The model under review builds one solid part; all positions refer to its coordinate system, in mm. A direction names the side the tool comes from. Coordinates: 2 decimals unless noted, no trailing zeros. Order: outer loops, then holes, each group sorted by start corner. A loop starts at its lowest first (then second) coordinate and runs counter-clockwise, first axis right, second up.
Autodesk Inventor part; units mm, degrees
ref_plane "YZ Plane" through (0, 0, 0) normal (1, 0, 0) x (0, 1, 0)
ref_plane "XZ Plane" through (0, 0, 0) normal (0, 1, 0) x (-1, 0, 0)
ref_plane "XY Plane" through (0, 0, 0) normal (0, 0, 1) x (1, 0, 0)
sketch "Náčrt1" plane through (0, 0, 0) normal (0, 0, 1) x (1, 0, 0)
  line L0 (-25, 0) -> (25, 0) construction
  line L1 (-25, -5) -> (25, -5)
  line L2 (25, 5) -> (-25, 5)
  arc A0 (-25, 5) -> (-25, -5) centre (-25, 0) ccw
  arc A1 (25, -5) -> (25, 5) centre (25, 0) ccw
  point P0 (0, 0)
  point P1 (30, 0)
  dimension "d0" = 30
  dimension "d1" = 5
extrude "Vysunutí1" add sketch "Náčrt1" along normal blind 0.5
sketch "Náčrt2" plane through (0, 0, 0) normal (0, 0, -1) x (-1, 0, 0)
  arc A0 (25, -5) -> (25, 5) centre (25, 0) ccw
  circle A1 centre (25, 0) radius 2
  point P0 (0, 0)
  dimension "d4" = 4
extrude "Vysunutí2" cut sketch "Náčrt2" against normal through all
pattern_linear "Obdélníkové pole1" count 7 spacing 10 along (1, 0, 0) of "Vysunutí2"
sketch "Náčrt3" plane through (0, 0, 0.5) normal (0, 0, 1) x (1, 0, 0)
  circle A0 centre (-15, 0) radius 2
  line L0 (-15, 2) -> (14.9898, 2)
  line L1 (14.9898, 2) -> (14.9898, -2)
  line L2 (14.9898, -2) -> (-15, -2)
  point P0 (0, 0)
extrude "Vysunutí3" cut sketch "Náčrt3" against normal blind 10 contours A0 L0 L1 L2
properties part number "2006"
(1) Consider section A-A (y = 0). Give the boundary of the cut face in (x, z), then the cut area to 3 significant figures.
(2) Tool access review of faces 5 (the face through (-0.4, 2.3, 0)), 6 (the face through (17, 0, 0.2)): name each direction out of +Z, -Z, +X, -X, +Y, -Y from which nothing blocks a thin tool from reaching the whole face with its end or side.
(3) Consider section B-B (z = 0.1). Give the number of separate pieces and of enclosed holes in the cut face, then the cut area to 3 significant figures.
(4) Wall thickness on line 1 (Y direction, x = -25, z = 0.45); line 2 (X direction, y = -0.25, z = 0.15); line 3 (X direction, y = -1.75, z = 0.4): over which ranges is each line inside the solid? List them lowest first.
(5) The part is to be moulded in two halves that separate along Y. For faces 1 (the face through (-17, 0, 0.2)), 2 (the face through (26.998, 0.088, 0.246)), 3 (the face through (-0.4, 2.3, 0.5)), 4 (the face through (-30, -0.1, 0.2)), say which applies: +Y half, -Y half, draft (parallel to the pull), parting line (faces both ways), or undercut.
(6) Consider section C-C (x = -4.5). Give the boundary of the cut face in (y, z).
(7) Consider section D-D (y = 3). Give the boundary of the cut face in (x, z), then the cut area to 3 significant figures.
Findings:
1. outline: (-30, 0) - (-27, 0) - (-27, 0.5) - (-30, 0.5) - close; (-23, 0) - (-17, 0) - (-17, 0.5) - (-23, 0.5) - close; (17, 0) - (23, 0) - (23, 0.5) - (17, 0.5) - close; (27, 0) - (30, 0) - (30, 0.5) - (27, 0.5) - close
1. area: 9.00 mm2
2. face 5: -Z, +X, -X, +Y, -Y
2. face 6: +Z, -Z
3. separate pieces: 1
3. enclosed holes: 3
3. area: 421 mm2
4. line 1: y = -5 to -2, 2 to 5
4. line 2: x = -29.99 to -26.98, -23.02 to -16.98, 16.98 to 23.02, 26.98 to 29.99
4. line 3: x = -29.68 to -25.97, -24.03 to -15.97, 15.97 to 24.03, 25.97 to 29.68
5. face 1: undercut
5. face 2: undercut
5. face 3: draft
5. face 4: parting line
6. outline: (-5, 0) - (-2, 0) - (-2, 0.5) - (-5, 0.5) - close; (2, 0) - (5, 0) - (5, 0.5) - (2, 0.5) - close
7. outline: (-29, 0) - (29, 0) - (29, 0.5) - (-29, 0.5) - close
7. area: 29.0 mm2
